Can you work these out from the model? Positions are in its coordinate system, mm. Face numbers are marked on the shaded views. A direction names the side the tool comes from. Coordinates: 2 decimals unless noted, no trailing zeros. Order: outer loops, then holes, each group sorted by start corner. A loop starts at its lowest first (then second) coordinate and runs counter-clockwise, first axis right, second up. Notation, with made-up numbers: (65, -24.75) -> (89, -24.75) arc R32 ccw to (89, 12.25) -> close; hole circle Ø2 at (86.25, 82). An arc over 180 degrees is marked (long way). Return JSON: item names as keys, results as strings. Group by question number.
1) For pin 1 (3 mm diameter, centred on x = -63.5, z = -13, fed in from +Y); pin 2 (15 mm diameter, centred on x = -60, z = -98, fed in from -Y); pin 3 (5 mm diameter, centred on x = 23.5, z = -18, fed in from +Y), each with a flat end and sliding along its axis, tell me the tip position at first contact or that it passes through.
2) If we section it at A-A, the plane z = -23: Please give me the cut outline in (x, y), then the cut area to 3 significant figures.
3) If we section it at D-D, the plane y = -3: Please give me the cut outline in (x, z).
4) Thinking about a two-plate mould opening in Z: for the marked faces 1, 2 and 3, which applies, +Z half, -Z half, draft (parallel to the pull), parting line (faces both ways), or undercut?
5) For the marked faces 4, 5, 6 and 7, which set-ups out of +Z, -Z, +X, -X, +Y, -Y let a thin tool reach every point of the face, with its end or its side?
6) If we section it at C-C, the plane x = 65: Please give me the cut outline in (y, z), then the cut area to 3 significant figures.
7) If I drill on probe 1 along X at (y, z) = (36, -15); probe 2 along X at (y, z) = (-13.5, -17); probe 3 along Y at (x, z) = (75, -23), over which ranges is the centre line in solid material (lowest first)? Write a range as from..to.
8) If we section it at B-B, the plane y = 28: Please give me the cut outline in (x, z).
from build123d import *

# Parameters (mm, degrees)
SKETCH1_W           = 160
SKETCH1_H           = 100
BOSS_EXTRUDE1_DEPTH = 126
SKETCH2_W           = 90
SKETCH2_H           = 60
CUT_EXTRUDE1_DEPTH  = 126
SKETCH3_R           = 5
CUT_EXTRUDE2_DEPTH  = 40
SHELL1_START        = -50
SHELL1_DEPTH        = 60
SHELL1_2_DEPTH      = 50
SHELL1_START_2      = 10
SHELL1_3_DEPTH      = 30
SKETCH4_W           = 20
SKETCH4_H           = 30
CUT_EXTRUDE3_DEPTH  = 180.655225362
FILLET1_R           = 5
SKETCH5_W           = 30
SKETCH5_H           = 20
CUT_EXTRUDE4_DEPTH  = 40
SKETCH6_W           = 110
SKETCH6_H           = 106
CUT_EXTRUDE5_DEPTH  = 10
SKETCH7_W           = 15
SKETCH7_H           = 73.639320226
CUT_EXTRUDE6_DEPTH  = 40
SKETCH8_R           = 5
CUT_EXTRUDE7_DEPTH  = 210.704554075


# Read off the part's stored shape, not the designer's step: Shell1
with BuildPart() as part:
    # Sketch1 → Boss-Extrude1 (new body)
    with BuildSketch(Plane.XY):
        Rectangle(SKETCH1_W, SKETCH1_H)
    extrude(amount=-BOSS_EXTRUDE1_DEPTH)

    # Sketch2 → Cut-Extrude1 (cut)
    with BuildSketch(Plane.XY):
        with Locations((0, 50)):
            Rectangle(SKETCH2_W, SKETCH2_H)
    extrude(amount=-CUT_EXTRUDE1_DEPTH, mode=Mode.SUBTRACT)

    # Sketch3 → Cut-Extrude2 (cut)
    with BuildSketch(Plane(origin=(0, 50, 0), x_dir=(1, 0, 0), z_dir=(0, 1, 0))):
        with Locations(Location((-65, 111, 0), (0, 0, 270))):
            Circle(SKETCH3_R)
        with Locations(Location((65, 111, 0), (0, 0, 90))):
            Circle(SKETCH3_R)
        with Locations(Location((65, 15, 0), (0, 0, 270))):
            Circle(SKETCH3_R)
        with Locations(Location((-65, 15, 0), (0, 0, 90))):
            Circle(SKETCH3_R)
    extrude(amount=-CUT_EXTRUDE2_DEPTH, mode=Mode.SUBTRACT)

    # Shell1 outline → Shell1 (cut)
    with BuildSketch(Plane(origin=(0, 0, 0), x_dir=(1, 0, 0), z_dir=(0, 1, 0)).offset(SHELL1_START)):
        with BuildLine():
            Line((70, 29.142135624), (70, 96.857864376))
            ThreePointArc((70, 96.857864376), (54.393398282, 100.393398282), (50.857864376, 116))
            Line((50.857864376, 116), (-50.857864376, 116))
            ThreePointArc((-50.857864376, 116), (-54.393398282, 100.393398282), (-70, 96.857864376))
            Line((-70, 96.857864376), (-70, 29.142135624))
            ThreePointArc((-70, 29.142135624), (-54.393398282, 25.606601718), (-50.857864376, 10))
            Line((-50.857864376, 10), (50.857864376, 10))
            ThreePointArc((50.857864376, 10), (54.393398282, 25.606601718), (70, 29.142135624))
        make_face()
    extrude(amount=SHELL1_DEPTH, mode=Mode.SUBTRACT)

    # Shell1 2 outline → Shell1 2 (cut)
    with BuildSketch(Plane(origin=(0, 0, 0), x_dir=(1, 0, 0), z_dir=(0, 1, 0)).offset(SHELL1_START)):
        with BuildLine():
            Line((50.857864376, 10), (70, 10))
            Line((70, 10), (70, 29.142135624))
            ThreePointArc((70, 29.142135624), (54.393398282, 25.606601718), (50.857864376, 10))
        make_face()
        with BuildLine():
            ThreePointArc((50.857864376, 116), (54.393398282, 100.393398282), (70, 96.857864376))
            Line((70, 96.857864376), (70, 116))
            Line((70, 116), (50.857864376, 116))
        make_face()
        with BuildLine():
            Line((-70, 10), (-50.857864376, 10))
            ThreePointArc((-50.857864376, 10), (-54.393398282, 25.606601718), (-70, 29.142135624))
            Line((-70, 29.142135624), (-70, 10))
        make_face()
        with BuildLine():
            ThreePointArc((-70, 96.857864376), (-54.393398282, 100.393398282), (-50.857864376, 116))
            Line((-50.857864376, 116), (-70, 116))
            Line((-70, 116), (-70, 96.857864376))
        make_face()
    extrude(amount=SHELL1_2_DEPTH, mode=Mode.SUBTRACT)

    # Shell1 3 outline → Shell1 3 (cut)
    with BuildSketch(Plane(origin=(0, 0, 0), x_dir=(1, 0, 0), z_dir=(0, 1, 0)).offset(SHELL1_START_2)):
        with BuildLine():
            ThreePointArc((55, 26.180339887), (62.094305849, 29.715873794), (70, 29.142135624))
            Line((70, 29.142135624), (70, 96.857864376))
            ThreePointArc((70, 96.857864376), (62.094305849, 96.284126206), (55, 99.819660113))
            Line((55, 99.819660113), (55, 26.180339887))
        make_face()
        with BuildLine():
            ThreePointArc((-70, 29.142135624), (-62.094305849, 29.715873794), (-55, 26.180339887))
            Line((-55, 26.180339887), (-55, 99.819660113))
            ThreePointArc((-55, 99.819660113), (-62.094305849, 96.284126206), (-70, 96.857864376))
            Line((-70, 96.857864376), (-70, 29.142135624))
        make_face()
    extrude(amount=SHELL1_3_DEPTH, mode=Mode.SUBTRACT)

    # Sketch4 → Cut-Extrude3 (cut, through all)
    with BuildSketch(Plane(origin=(0, 50, 0), x_dir=(1, 0, 0), z_dir=(0, 1, 0))):
        with Locations((0, 90)):
            Rectangle(SKETCH4_W, SKETCH4_H)
        with Locations((0, 36)):
            Rectangle(SKETCH4_W, SKETCH4_H)
    extrude(amount=-CUT_EXTRUDE3_DEPTH, mode=Mode.SUBTRACT)

    # Fillet1
    fillet1_edges = [part.edges().sort_by_distance(p)[0] for p in [
        (-10, 15, -21),
        (-10, 15, -51),
        (10, 15, -51),
        (10, 15, -21),
        (10, 15, -105),
        (10, 15, -75),
        (-10, 15, -75),
        (-10, 15, -105),
    ]]
    fillet(fillet1_edges, radius=FILLET1_R)

    # Sketch5 → Cut-Extrude4 (cut)
    with BuildSketch(Plane(origin=(0, 0, -126), x_dir=(-1, 0, 0), z_dir=(0, 0, -1))):
        with Locations((-65, -10)):
            Rectangle(SKETCH5_W, SKETCH5_H)
        with Locations((65, -10)):
            Rectangle(SKETCH5_W, SKETCH5_H)
    extrude(amount=-CUT_EXTRUDE4_DEPTH, mode=Mode.SUBTRACT)

    # Sketch6 → Cut-Extrude5 (cut)
    with BuildSketch(Plane.XZ.offset(-10)):
        with Locations((0, -63)):
            Rectangle(SKETCH6_W, SKETCH6_H)
    extrude(amount=CUT_EXTRUDE5_DEPTH, mode=Mode.SUBTRACT)

    # Sketch7 → Cut-Extrude6 (cut)
    with BuildSketch(Plane.XZ.offset(-40)):
        with Locations((-62.5, -63)):
            Rectangle(SKETCH7_W, SKETCH7_H)
    cut_extrude6 = extrude(amount=CUT_EXTRUDE6_DEPTH, mode=Mode.SUBTRACT)

    # Mirror1: Cut-Extrude6 across plane
    add(cut_extrude6.mirror(Plane(origin=(0, 0, 0), x_dir=(0, 0, 1), z_dir=(1, 0, 0))), mode=Mode.SUBTRACT)

    # Sketch8 → Cut-Extrude7 (cut, through all)
    with BuildSketch(Plane(origin=(80, 0, 0), x_dir=(0, 0, -1), z_dir=(1, 0, 0))):
        with Locations((23, -20)):
            Circle(SKETCH8_R)
    extrude(amount=-CUT_EXTRUDE7_DEPTH, mode=Mode.SUBTRACT)


solid = part.part
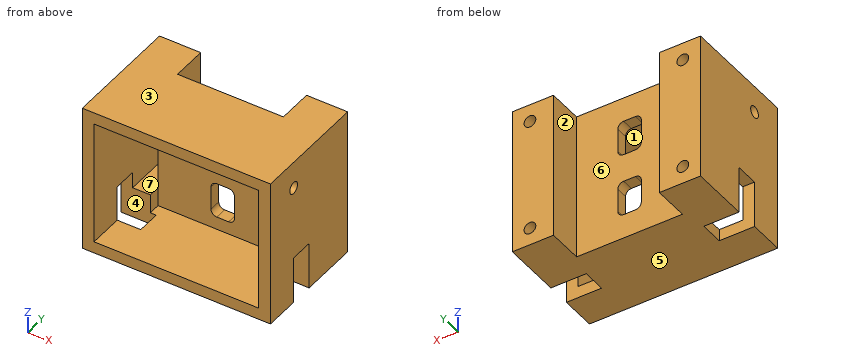
Result sheet:
{
 "1": {"pin 1": "stops at y = 10", "pin 2": "stops at y = 0", "pin 3": "stops at y = 20"},
 "2": {"outline": "(-80, -50) -> (-70, -50) -> (-70, -25) -> (-80, -25) -> close; (-80, -15) -> (-70, -15) -> (-70, 0) -> (-55, 0) -> (-55, 10) -> (-9, 10) -> (-9, 20) -> (-45, 20) -> (-45, 50) -> (-80, 50) -> close; (9, 10) -> (55, 10) -> (55, 0) -> (70, 0) -> (70, -15) -> (80, -15) -> (80, 50) -> (45, 50) -> (45, 20) -> (9, 20) -> close; (70, -50) -> (80, -50) -> (80, -25) -> (70, -25) -> close", "area": "4,820 mm2"},
 "3": {"outline": "(-80, -86) -> (-70, -86) -> (-70, -10) -> (70, -10) -> (70, -86) -> (80, -86) -> (80, 0) -> (-80, 0) -> close; (-50, -126) -> (50, -126) -> (50, -116) -> (-50, -116) -> close"},
 "4": {"face 1": "undercut", "face 2": "draft", "face 3": "+Z half"},
 "5": {"face 4": "-Z, -X", "face 5": "-Z, +X, -X, +Y, -Y", "face 6": "+Z, -Z, +Y", "face 7": "-Y"},
 "6": {"outline": "(-50, -126) -> (-20, -126) -> (-20, -116) -> (-50, -116) -> close; (-50, -10) -> (0, -10) -> (0, -26.18) -> (40, -26.18) -> (40, -99.82) -> (0, -99.82) -> (0, -126) -> (50, -126) -> (50, -116) -> (10, -116) -> (10, -106) -> (50, -106) -> (50, -20) -> (10, -20) -> (10, -10) -> (50, -10) -> (50, 0) -> (-50, 0) -> close", "area": "3,350 mm2"},
 "7": {"probe 1": "x = -80..-70, -60..-45, 45..60, 70..80", "probe 2": "x = -80..-70, 70..80", "probe 3": "y = -50..-25, -15..50"},
 "8": {"outline": "(-80, -126) -> (-45, -126) -> (-45, 0) -> (-80, 0) -> close; (45, -126) -> (80, -126) -> (80, 0) -> (45, 0) -> close; hole circle Ø10 at (-65, -111); hole (-70, -99.82) -> (-55, -99.82) -> (-55, -26.18) -> (-70, -26.18) -> close; hole circle Ø10 at (-65, -15); hole (55, -99.82) -> (70, -99.82) -> (70, -26.18) -> (55, -26.18) -> close; hole circle Ø10 at (65, -111); hole circle Ø10 at (65, -15)"}
}
